Design review of the part built by this model. Coordinates are the model's own, in mm. Face numbers are marked on the shaded views. A direction names the side the tool comes from. Coordinates: 2 decimals unless noted, no trailing zeros. Write each loop counter-clockwise with the first axis right and the second up, starting at its lowest first coordinate (ties: lowest second). Pieces come first, ordered by that corner, then holes.
Q1. The part is to be moulded in two halves that separate along Z. For the marked faces 3, 4 and 5, say which applies: released by +Z, released by -Z, zero draft, split by the parting line, or undercut.
Q2. Take a section at C-C, the plane x = 0. Write out the cut boundary in (y, z) (3 decimals).
Q3. For L1, parallel to Z at x = 1, y = -10; L2, parallel to Z at x = 29, y = -13; L3, parallel to Z at x = -4.5, y = -11.25, list the stretches that pass through material, from the lowest coordinate up.
Q4. For the marked faces 1 and 2, list the 3-axis set-ups (+Z, -Z, +X, -X, +Y, -Y) from which the entire face can be reached by the end or side of a thin tool; tool diameter is ignored.
Q5. Take a section at A-A, the plane z = 48.5. Write out the cut boundary in (x, y), plus the area to 3 significant figures.
Q6. Take a section at B-B, the plane z = 101.6. Write out the cut boundary in (x, y) (3 decimals).
Q7. For pin 1 Ø9 at (x, z) = (22, 68) entering from +Y; pin 2 Ø5 at (y, z) = (-13, 53) entering from -X; pin 3 Ø10 at (y, z) = (-5, -12.5) entering from +X, all flat-tipped, find the tip position at first contact; note any pin that passes through.
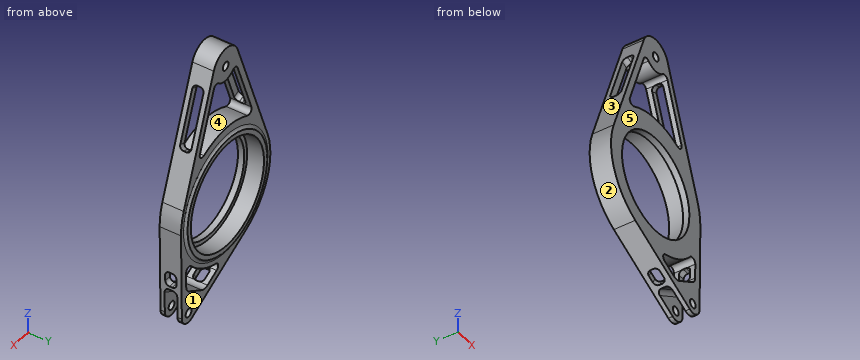
from build123d import *

# Parameters (mm, degrees)
SKETCH1_R           = 36.800037017
SKETCH1_R_2         = 3.175
BOSS_EXTRUDE1_DEPTH = 16.002
SKETCH5_R           = 43.561
SKETCH5_R_2         = 40.000036967
BOSS_EXTRUDE3_DEPTH = 1.27
SKETCH6_R           = 40.000036967
SKETCH6_R_2         = 36.800037017
CUT_EXTRUDE2_DEPTH  = 11.3284
FILLET2_R           = 3.175
CUT_EXTRUDE3_DEPTH  = 4.7625
CUT_EXTRUDE4_DEPTH  = 18.80616
FILLET3_R           = 3.175
FILLET5_R           = 6.35
CUT_EXTRUDE5_REACH  = 140.003
SKETCH22_W          = 44.42320982
SKETCH22_H          = 8.382
CUT_EXTRUDE6_REACH  = 140.003
SKETCH23_W          = 44.42320982
SKETCH23_H          = 8.382
CUT_EXTRUDE7_REACH  = 154.858
SKETCH24_W          = 11.166222722
SKETCH24_H          = 8.382
CUT_EXTRUDE8_REACH  = 177.085
SKETCH25_W          = 11.166222722
SKETCH25_H          = 8.382
FILLET6_R           = 3.175


with BuildPart() as part:
    # Sketch1 → Boss-Extrude1 (new body)
    with BuildSketch(Plane(origin=(0, 0, 0), x_dir=(1, 0, 0), z_dir=(0, 1, 0))):
        with BuildLine():
            Line((-45.845642474, -16.794270915), (-13.030803906, -106.373471135))
            ThreePointArc((-13.030803906, -106.373471135), (0, -115.477603436), (13.030803906, -106.373471135))
            Line((13.030803906, -106.373471135), (45.845642474, -16.794270915))
            ThreePointArc((45.845642474, -16.794270915), (48.13062155, -8.204495023), (48.820472847, 0.657191296))
            Line((48.820472847, 0.657191296), (47.919430717, 67.592500854))
            ThreePointArc((47.919430717, 67.592500854), (44.347868478, 73.807247594), (37.183825898, 74.043103011))
            Line((37.183825898, 74.043103011), (-22.33955821, 43.414451608))
            ThreePointArc((-22.33955821, 43.414451608), (-45.481622278, 17.756477815), (-45.845642474, -16.794270915))
        make_face()
        with Locations(Location((0, 0, 0), (0, 0, 270))):
            Circle(SKETCH1_R, mode=Mode.SUBTRACT)
        with Locations(Location((0, -101.6, 0), (0, 0, 270))):
            Circle(SKETCH1_R_2, mode=Mode.SUBTRACT)
        with Locations(Location((40.554098018, 67.493353257, 0), (0, 0, 270))):
            Circle(SKETCH1_R_2, mode=Mode.SUBTRACT)
    extrude(amount=BOSS_EXTRUDE1_DEPTH)

    # Sketch5 → Boss-Extrude3 (add)
    with BuildSketch(Plane.XZ):
        with Locations(Location((0, 0, 0), (0, 0, 90))):
            Circle(SKETCH5_R)
        with Locations(Location((0, 0, 0), (0, 0, 270))):
            Circle(SKETCH5_R_2, mode=Mode.SUBTRACT)
    extrude(amount=BOSS_EXTRUDE3_DEPTH)

    # Sketch6 → Cut-Extrude2 (cut)
    with BuildSketch(Plane.XZ):
        with Locations(Location((0, 0, 0), (0, 0, 270))):
            Circle(SKETCH6_R)
        with Locations(Location((0, 0, 0), (0, 0, 270))):
            Circle(SKETCH6_R_2, mode=Mode.SUBTRACT)
    extrude(amount=-CUT_EXTRUDE2_DEPTH, mode=Mode.SUBTRACT)

    # Fillet2
    # the kernel refuses this fillet: 3.175 mm, written as the material it adds along each edge
    with BuildSketch(Plane(origin=(0, 0, 0), x_dir=(0, 0, 1), z_dir=(1, 0, 0))) as fillet2_piece_1:
        with BuildLine():
            CenterArc((46.101, 3.175), FILLET2_R, 216.869897646, 53.130102354)
            Line((46.101, 0), (46.101, -0.0635))
            Line((46.101, -0.0635), (43.561, -0.0635))
            Line((43.561, -0.0635), (43.4975, 0))
            ThreePointArc((43.4975, 0), (43.4975, 0.635), (43.5102, 1.2319))
            Line((43.5102, 1.2319), (43.561, 1.27))
        make_face()
    revolve(axis=Axis((0, 0, 0), (0, -1, 0)))

    # Sketch7 → Cut-Extrude3 (cut, symmetric)
    with BuildSketch(Plane(origin=(0, 8.001, 0), x_dir=(-1, 0, 0), z_dir=(0, -1, 0))):
        Polygon((-8.642366299, 86.667856133), (-2.101382747, 75.781831414), (-66.916726186, 36.836844033), (-73.457709737, 47.722868752), (-97.309602446, 87.419084403), (-32.494259008, 126.364071784), align=None)
    extrude(amount=CUT_EXTRUDE3_DEPTH, both=True, mode=Mode.SUBTRACT)


with BuildPart() as body_2:
    # Mirror1: mirrored copy
    add(part.part.mirror(Plane(origin=(0, -1.27, 0), x_dir=(0, 0, 1), z_dir=(0, -1, 0))))

    # Sketch9 → Cut-Extrude4 (cut)
    with BuildSketch(Plane(origin=(0, 0, 0), x_dir=(1, 0, 0), z_dir=(0, 1, 0))):
        with BuildLine():
            Line((22.973751547, 61.018010354), (43.090182322, 48.930839307))
            Line((43.090182322, 48.930839307), (43.428261446, 23.816108157))
            ThreePointArc((43.428261446, 23.816108157), (25.50983585, 42.455496404), (0.640041598, 49.525864422))
            Line((0.640041598, 49.525864422), (22.973751547, 61.018010354))
        make_face()
        with BuildLine():
            Line((-31.360879833, -41.566574505), (-10.770746379, -97.774307586))
            ThreePointArc((-10.770746379, -97.774307586), (0, -90.17), (10.770746379, -97.774307586))
            Line((10.770746379, -97.774307586), (31.360879833, -41.566574505))
            ThreePointArc((31.360879833, -41.566574505), (0, -52.07), (-31.360879833, -41.566574505))
        make_face()
    extrude(amount=-CUT_EXTRUDE4_DEPTH, mode=Mode.SUBTRACT)

    # Fillet3
    fillet3_edges = [body_2.edges().sort_by_distance(p)[0] for p in [
        (0.640041598, -10.541, -49.525864422),
        (43.428261446, -10.541, -23.816108157),
        (-31.360879833, -10.541, 41.566574505),
        (31.360879833, -10.541, 41.566574505),
        (10.770746379, -10.541, 97.774307586),
        (-10.770746379, -10.541, 97.774307586),
        (34.013114467, -15.3035, -56.607328538),
        (34.013114467, -5.7785, -56.607328538),
    ]]
    fillet(fillet3_edges, radius=FILLET3_R)

    # Fillet5
    fillet5_edges = [body_2.edges().sort_by_distance(p)[0] for p in [
        (22.973751547, -10.541, -61.018010354),
        (43.090182322, -10.541, -48.930839307),
    ]]
    fillet(fillet5_edges, radius=FILLET5_R)

    # Sketch22 → Cut-Extrude5 (cut, up to next)
    with BuildSketch(Plane(origin=(45.845642474, 0, 16.794270915), x_dir=(0.34396941500000017, 0, -0.9389808525974094), z_dir=(0.9389808525974093, 0, 0.3439694150000001)), mode=Mode.PRIVATE) as cut_extrude5_sk1:
        with Locations((-59.709519033, -10.541)):
            Rectangle(SKETCH22_W, SKETCH22_H)
    cut_extrude5_tool1 = extrude(cut_extrude5_sk1.sketch, amount=-CUT_EXTRUDE5_REACH, mode=Mode.PRIVATE) & body_2.part
    add(cut_extrude5_tool1.solids().sort_by_distance((25.307394, -10.541, 72.860366))[0], mode=Mode.SUBTRACT)

    # Sketch23 → Cut-Extrude6 (cut, up to next)
    with BuildSketch(Plane(origin=(-45.845642474, 0, 16.794270915), x_dir=(0.3439694150000003, 0, 0.9389808525974093), z_dir=(-0.9389808525974094, 0, 0.34396941500000033)), mode=Mode.PRIVATE) as cut_extrude6_sk1:
        with Locations((59.709519033, -10.541)):
            Rectangle(SKETCH23_W, SKETCH23_H)
    cut_extrude6_tool1 = extrude(cut_extrude6_sk1.sketch, amount=-CUT_EXTRUDE6_REACH, mode=Mode.PRIVATE) & body_2.part
    add(cut_extrude6_tool1.solids().sort_by_distance((-25.307394, -10.541, 72.860366))[0], mode=Mode.SUBTRACT)

    # Sketch24 → Cut-Extrude7 (cut, up to next)
    with BuildSketch(Plane(origin=(48.820472847, 0, -0.657191296), x_dir=(-0.01346016787133038, 0, -0.9999094078369678), z_dir=(0.9999094078369678, 0, -0.01346016787133038)), mode=Mode.PRIVATE) as cut_extrude7_sk1:
        with Locations((39.22684129, -10.541)):
            Rectangle(SKETCH24_W, SKETCH24_H)
    cut_extrude7_tool1 = extrude(cut_extrude7_sk1.sketch, amount=-CUT_EXTRUDE7_REACH, mode=Mode.PRIVATE) & body_2.part
    add(cut_extrude7_tool1.solids().sort_by_distance((48.292473, -10.541, -39.880479))[0], mode=Mode.SUBTRACT)

    # Sketch25 → Cut-Extrude8 (cut, up to next)
    with BuildSketch(Plane(origin=(-22.33955821, 0, -43.414451608), x_dir=(-0.8891867707725541, 0, 0.4575444095200786), z_dir=(-0.4575444095200785, 0, -0.889186770772554)), mode=Mode.PRIVATE) as cut_extrude8_sk1:
        with Locations((-39.22684129, -10.541)):
            Rectangle(SKETCH25_W, SKETCH25_H)
    cut_extrude8_tool1 = extrude(cut_extrude8_sk1.sketch, amount=-CUT_EXTRUDE8_REACH, mode=Mode.PRIVATE) & body_2.part
    add(cut_extrude8_tool1.solids().sort_by_distance((12.54043, -10.541, -61.362474))[0], mode=Mode.SUBTRACT)

    # Fillet6
    fillet6_edges = [body_2.edges().sort_by_distance(p)[0] for p in [
        (15.28227003, -14.732, 92.842955406),
        (15.28227003, -6.35, 92.842955406),
        (30.562495524, -6.35, 51.130411974),
        (30.562495524, -14.732, 51.130411974),
        (-30.562495524, -14.732, 51.130411974),
        (-30.562495524, -6.35, 51.130411974),
        (-15.28227003, -6.35, 92.842955406),
        (-15.28227003, -14.732, 92.842955406),
        (45.827852698, -14.732, -34.263684541),
        (45.827852698, -6.35, -34.263684541),
        (45.677553466, -6.35, -45.428895691),
        (45.677553466, -14.732, -45.428895691),
        (18.667021686, -14.732, -61.658460536),
        (18.667021686, -6.35, -61.658460536),
        (8.738164162, -6.35, -56.549417754),
        (8.738164162, -14.732, -56.549417754),
    ]]
    fillet(fillet6_edges, radius=FILLET6_R)


solid = body_2.part
Responses:
1. face 3: released by +Z
1. face 4: undercut
1. face 5: zero draft
2. outline: (-18.542, -54.91) - (-2.54, -54.91) - (-2.54, -46.101) arc R3.175 cw to (-1.27, -43.561) - (-1.27, -40) - (-13.868, -40) - (-13.868, -36.8) - (-18.542, -36.8) - close; (-18.542, 36.8) - (-13.868, 36.8) - (-13.868, 40) - (-1.27, 40) - (-1.27, 43.561) arc R3.175 cw to (-2.54, 46.101) - (-2.54, 52.07) - (-18.542, 52.07) - close; (-18.542, 90.17) - (-2.54, 90.17) - (-2.54, 98.425) - (-18.542, 98.425) - close; (-18.542, 104.775) - (-2.54, 104.775) - (-2.54, 115.478) - (-18.542, 115.478) - close
3. L1: z = -55.42 to -39.99, 39.99 to 52.06, 90.21 to 98.59, 104.61 to 115.44
3. L2: z = -59.76 to -57.4, -40.15 to -27.55, 27.55 to 50.93
3. L3: z = -52.59 to -39.75, 39.75 to 51.88, 91.09 to 114.73
4. face 1: +Y
4. face 2: -X, +Y, -Y
5. outline: (-34.23, -18.54) - (-28.3, -18.54) - (-28.3, -2.54) - (-34.23, -2.54) - close; (-18.95, -18.54) - (18.95, -18.54) - (18.95, -2.54) - (-18.95, -2.54) - close; (28.3, -18.54) - (34.23, -18.54) - (34.23, -2.54) - (28.3, -2.54) - close
5. area: 796 mm2
6. outline: (-14.779, -18.542) - (-3.175, -18.542) - (-3.175, -2.54) - (-14.779, -2.54) - close; (3.175, -18.542) - (14.779, -18.542) - (14.779, -2.54) - (3.175, -2.54) - close
7. pin 1: stops at y = -2.54
7. pin 2: stops at x = -33.5
7. pin 3: stops at x = 48.73
